```python
from build123d import *

# Parameters (mm, degrees)
BOSS_EXTRUDE1_DEPTH = 120
BOSS_EXTRUDE2_DEPTH = 26.917181
CUT_EXTRUDE3_DEPTH  = 34.246933562
SKETCH7_R           = 1.55
CUT_EXTRUDE4_DEPTH  = 10
CUT_EXTRUDE5_DEPTH  = 4
FILLET1_R           = 50
SKETCH10_R          = 1.5
CUT_EXTRUDE6_DEPTH  = 40.591109915
CHAMFER4_SIZE       = 3.5
SKETCH12_R          = 4
CUT_EXTRUDE8_DEPTH  = 5
SKETCH12_3_R        = 4
CUT_EXTRUDE9_DEPTH  = 9


with BuildPart() as part:
    # Sketch1 → Boss-Extrude1 (new body)
    with BuildSketch(Plane.XY):
        Polygon((12, 26), (5.033320997, 0), (22.41998587, -4.658742812), (29.386664873, 21.341257188), align=None)
        Polygon((0, 0), (0, 26), (12, 26), (5.033320997, 0), align=None)
    extrude(amount=-BOSS_EXTRUDE1_DEPTH)

    # Sketch3 → Boss-Extrude2 (add)
    with BuildSketch(Plane(origin=(7.303847577, 27.258330249, 0), x_dir=(0.965925826, -0.258819045, 0), z_dir=(0.258819045, 0.965925826, 0))):
        Polygon((22.861814743, 0), (32.861814743, 52.5), (32.861814743, 67.5), (22.861814743, 120), align=None)
    extrude(amount=-BOSS_EXTRUDE2_DEPTH)

    # Sketch6 → Cut-Extrude3 (cut, through all)
    with BuildSketch(Plane(origin=(0, 26, 0), x_dir=(1, 0, 0), z_dir=(0, 1, 0))):
        Polygon((0, 100), (7, 93), (7, 27), (0, 20), align=None)
    extrude(amount=-CUT_EXTRUDE3_DEPTH, mode=Mode.SUBTRACT)

    # Sketch7 → Cut-Extrude4 (cut)
    with BuildSketch(Plane.ZY):
        with Locations((-110, 15)):
            Circle(SKETCH7_R)
        with Locations((-10, 15)):
            Circle(SKETCH7_R)
    extrude(amount=-CUT_EXTRUDE4_DEPTH, mode=Mode.SUBTRACT)

    # Sketch8 → Cut-Extrude5 (cut)
    with BuildSketch(Plane.ZY.offset(-5)):
        Polygon((-113, 16.732050808), (-113, 26), (-107, 26), (-107, 16.732050808), (-107, 13.267949192), (-110, 11.535898385), (-113, 13.267949192), align=None)
        Polygon((-13, 26), (-13, 16.732050808), (-13, 13.267949192), (-10, 11.535898385), (-7, 13.267949192), (-7, 16.732050808), (-7, 26), align=None)
    extrude(amount=-CUT_EXTRUDE5_DEPTH, mode=Mode.SUBTRACT)

    # Fillet1
    fillet1_edges = [part.edges().sort_by_distance(p)[0] for p in [
        (35.562583594, 5.753066588, -52.5),
        (35.562583594, 5.753066588, -67.5),
    ]]
    fillet(fillet1_edges, radius=FILLET1_R)

    # Sketch10 → Cut-Extrude6 (cut, through all)
    with BuildSketch(Plane(origin=(31.742075559, -8.505263512, 0), x_dir=(0, 0, -1), z_dir=(0.965925826, -0.258819045, 0))):
        with Locations((60, 22.261309679)):
            Circle(SKETCH10_R)
        with Locations((60, 7.261309679)):
            Circle(SKETCH10_R)
    extrude(amount=-CUT_EXTRUDE6_DEPTH, mode=Mode.SUBTRACT)

    # Chamfer4
    chamfer4_edges = [part.edges().sort_by_distance(p)[0] for p in [
        (20.693332437, 23.670628594, -120),
        (20.693332437, 23.670628594, 0),
    ]]
    chamfer(chamfer4_edges, length=CHAMFER4_SIZE)

    # Sketch12 → Cut-Extrude8 (cut)
    with BuildSketch(Plane(origin=(-2.065328361, 0.553403067, 0), x_dir=(0, 0, -1), z_dir=(0.965925826, -0.258819045, 0))):
        with Locations((60, 22.261309679)):
            Circle(SKETCH12_R)
    extrude(amount=CUT_EXTRUDE8_DEPTH, mode=Mode.SUBTRACT)

    # Sketch12<3> → Cut-Extrude9 (cut)
    with BuildSketch(Plane(origin=(-2.065328361, 0.553403067, 0), x_dir=(0, 0, -1), z_dir=(0.965925826, -0.258819045, 0))):
        with Locations((60, 7.261309679)):
            Circle(SKETCH12_3_R)
    extrude(amount=CUT_EXTRUDE9_DEPTH, mode=Mode.SUBTRACT)


solid = part.part
```
Read the model definition and answer for the solid it produces. Units are mm, in the model's axes. A direction names the side the tool comes from. Coordinates: 2 decimals unless noted, no trailing zeros. Loops run counter-clockwise (first coordinate to the right, second up) from the corner with the lowest first, then second, coordinate; pieces in that order, holes last.
(1) A tool of negligible diameter and unlimited length cuts with its end or side. For faces 4 (the face through (3, 0, -107)), 5 (the face through (7, 20, -13)), 6 (the face through (7, 13, -60)), 7 (the face through (9.493, 16.537, -10.202)), 8 (the face through (8.52, 9.34, -59.48)), from which of +Z, -Z, +X, -X, +Y, -Y can it reach the whole face along a straight path? Write none if from no direction.
Solution:
face 4: +Z, -Z, -X, -Y
face 5: +Y
face 6: -X, +Y, -Y
face 7: -X
face 8: none
(2) The mould has two halves that part along X. Classify faces 1 (the face through (7, 20, -7)), 2 (the face through (9.49, 15.07, -111.55)), 3 (the face through (30.294, 7.36, -23.597)): released by +X, released by -X, zero draft, split by the parting line, or undercut.
Solution:
face 1: undercut
face 2: zero draft
face 3: released by +X
(3) The part is cut by section B-B (z = -85). Determine the outline of the cut face in (x, y), and give its area (3 significant figures).
Solution:
outline: (7, -0.53) - (28.86, -6.38) - (35.83, 19.62) - (12, 26) - (7, 26) - close
area: 703 mm2
(4) Flat-ended cylindrical pins translate along their axes: pin 1 Ø8 at (x, z) = (17, -103.5) entering from +Y; pin 2 Ø5 at (y, z) = (15, -110) entering from +X; pin 3 Ø3 at (y, z) = (15, -110) entering from -X. Find the tip coordinate at first contact, or state that the pin passes through.
Solution:
pin 1: stops at y = 25.73
pin 2: stops at x = 30.49
pin 3: stops at x = 10
(5) The part is cut by section A-A (y = 23.5). Count the separate pieces of the cut face and the enclosed holes in it, and give its area (3 significant figures).
Solution:
separate pieces: 1
enclosed holes: 2
area: 1,940 mm2
(6) Consider line 1 along Y through (x, z) = (27.5, -59); line 2 along Z through (x, y) = (5.5, 13.5); line 3 along Y through (x, z) = (9.45, -110). Determine where each line is inside the solid, lowest interval first.
Solution:
line 1: y = -6.02 to -1.01, 1.31 to 14.52, 16.84 to 21.85
line 2: z = -120 to -113, -107 to -94.5, -25.5 to -13, -7 to 0
line 3: y = -1.18 to 13.45, 16.55 to 26
